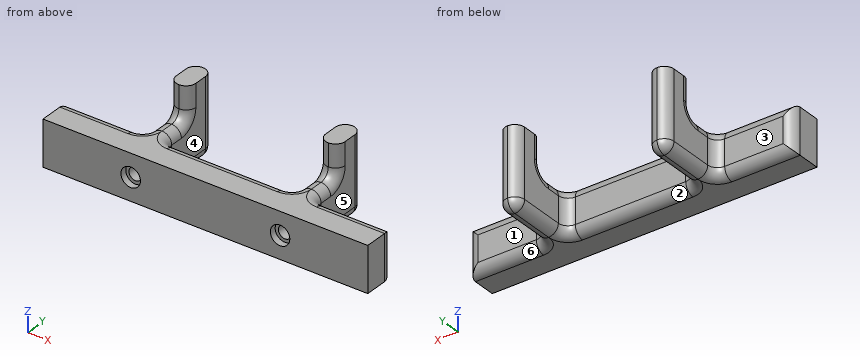
```python
from build123d import *

# Parameters (mm, degrees)
F0_W           = 30
F0_H           = 100
F1_DEPTH       = 70
F2_W           = 30
F2_H           = 50
F3_DEPTH       = 50
F4_F1_R        = 15
F4_F2_R        = 14.9999
F6_D           = 20
F6_DEPTH       = 50
F6_CBORE_D     = 30
F6_CBORE_DEPTH = 10
F6_TIP         = 6.0086061903


# Not quite as in the source:
# - a fillet or chamfer is up to 0.001 mm smaller than in the source, because OpenCascade refuses the exact size


with BuildPart() as f1:
    # F0 (on Top) → F1 (new body)
    with BuildSketch(Plane.XY):
        Polygon((-130, 0), (-250, 0), (-250, -50), (250, -50), (250, 0), (130, 0), (100, 0), (-100, 0), align=None)
        with Locations((-115, 50)):
            Rectangle(F0_W, F0_H)
        with Locations((115, 50)):
            Rectangle(F0_W, F0_H)
    extrude(amount=F1_DEPTH)

    # F2 (on face) → F3 (join)
    with BuildSketch(Plane.XY.offset(70)):
        with Locations((-115, 75)):
            Rectangle(F2_W, F2_H)
        with Locations((115, 75)):
            Rectangle(F2_W, F2_H)
    extrude(amount=F3_DEPTH)

    # F4: fillet of radius 15 on 24 edges, made by hand

    # F4_f1
    f4_f1_edges = [f1.edges().sort_by_distance(p)[0] for p in [
        (-115, 50, 70),
        (115, 50, 70),
        (100, 0, 35),
        (-130, 0, 35),
        (-100, 0, 35),
        (130, 0, 35),
    ]]
    fillet(f4_f1_edges, radius=F4_F1_R)

    # F4_f2 (radius 15 in the source; OpenCascade refuses exactly that, so slightly less here)
    f4_f2_edges = [f1.edges().sort_by_distance(p)[0] for p in [
        (-197.5, 0, 70),
        (115, 100, 0),
        (197.5, 0, 0),
        (197.5, 0, 70),
        (250, 0, 35),
        (130, 100, 60),
        (100, 100, 60),
        (-197.5, 0, 0),
        (-250, 0, 35),
        (-100, 100, 60),
        (-115, 100, 0),
        (-130, 100, 60),
        (0, 0, 70),
        (130, 57.5, 0),
        (100, 57.5, 0),
        (0, 0, 0),
        (-100, 57.5, 0),
        (-130, 57.5, 0),
        (-134.3933982822, 4.3933982822, 0),
        (-95.6066017178, 4.3933982822, 0),
        (95.6066017178, 4.3933982822, 0),
        (134.3933982822, 4.3933982822, 0),
        (95.6066017178, 4.3933982822, 70),
        (-95.6066017178, 4.3933982822, 70),
        (134.3933982822, 4.3933982822, 70),
        (-134.3933982822, 4.3933982822, 70),
    ]]
    fillet(f4_f2_edges, radius=F4_F2_R)

    # F6
    with Locations(Plane.XZ.offset(50)):
        with Locations((-114.9999999844, 35), (115.0000000156, 35)):
            CounterBoreHole(F6_D / 2, F6_CBORE_D / 2, F6_CBORE_DEPTH, depth=F6_DEPTH)
            with Locations((0, 0, -(F6_DEPTH + F6_TIP / 2))):  # 118° drill point
                Cone(0, F6_D / 2, F6_TIP, mode=Mode.SUBTRACT)


solid = f1.part
```
Work out the finished part from the listing and answer in its coordinate system (mm). Face numbers are marked on the shaded views. A direction names the side the tool comes from. Give positions to 0.01 mm unless a question says otherwise; leave off trailing zeros. Write each loop counter-clockwise with the first axis right and the second up, starting at its lowest first coordinate (ties: lowest second). Pieces come first, ordered by that corner, then holes.
(1) The part is cut by section C-C on y = -9. Count the separate pieces of the cut face and the enclosed holes in it, plus the area to 3 significant figures.
Final values:
separate pieces: 1
enclosed holes: 2
area: 33,200 mm2
(2) Which of the six approach directions +Z, -Z, +X, -X, +Y, -Y give full straight-line access (tool end or side, diameter ignored) to the marked faces 1, 2 and 3?
Final values:
face 1: +Z, -Z, +X, +Y
face 2: -Z, +Y
face 3: +Z, -Z, -X, +Y
(3) Straight lines are drawn through the part: line 1 (Z direction, x = 115, y = -12); line 2 (X direction, y = 36.5, z = 55); line 3 (Z direction, x = 115, y = -43). For each, find the intervals that lie inside material, in ascending order.
Final values:
line 1: z = 0 to 25, 45 to 70
line 2: x = -130 to -100, 100 to 130
line 3: z = 0 to 20, 50 to 70
(4) The mould has two halves that part along X. Classify the marked faces 4, 5 and 6: pulls with the +X half, pulls with the -X half, needs draft (parallel to the pull), parting line crosses it, or undercut.
Final values:
face 4: undercut
face 5: pulls with the +X half
face 6: needs draft
(5) Flat-ended cylindrical pins translate along their axes: pin 1 Ø10 at (x, y) = (-34.5, -15.5) entering from +Z; pin 2 Ø4 at (x, z) = (122.5, 104.5) entering from -Y; pin 3 Ø23 at (x, z) = (115, 35) entering from -Y. Find the tip coordinate at first contact, or state that the pin passes through.
Final values:
pin 1: stops at z = 70
pin 2: stops at y = 51.04
pin 3: stops at y = -40
(6) The part is cut by section B-B on x = -63. Write down the section's boundary in (y, z), plus the area to 3 significant figures.
Final values:
outline: (-50, 0) - (-15, 0) arc R15 ccw to (0, 15) - (0, 55) arc R15 ccw to (-15, 70) - (-50, 70) - close
area: 3,400 mm2
